The listing builds one solid part. Answer for the finished solid, in the listing's coordinates (mm). Face numbers are marked on the shaded views. A direction names the side the tool comes from. Give positions to 0.01 mm unless a question says otherwise; leave off trailing zeros. Write each loop counter-clockwise with the first axis right and the second up, starting at its lowest first coordinate (ties: lowest second). Pieces come first, ordered by that corner, then holes. Notation, with made-up numbers: (-13, 52.5) - (20, 52.5) arc R23 cw to (20, 86.5) - close; hole circle Ø1 at (-4, 86.25). An arc over 180 degrees is marked (long way). Answer as CSV lines item,"result". Start each with the question number.
(1) For the marked faces 1, 2 and 3, determine the directions among +Z, -Z, +X, -X, +Y, -Y from which every point of the face is accessible in a straight line to the end or side of a thin tool.
(2) Each of these flat-tipped pins is pushed along its axis until it touches: pin 1 Ø5 at (y, z) = (30.5, 10.5) entering from +X; pin 2 Ø1.3 at (x, y) = (-1, 28) entering from +Z; pin 3 Ø5 at (y, z) = (13.5, 3) entering from -X. Where does it stop, or does it pass through?
(3) Find section D-D (y = 7). Write down the section's boundary in (x, z), then the cut area to 3 significant figures.
(4) Find section B-B (x = 25). Write down the section's boundary in (y, z).
(5) Straight lines are drawn through the part: probe 1 along Y at (x, z) = (-25, 6.25); probe 2 along Y at (x, z) = (0, 7.5); probe 3 along Y at (x, z) = (-30, 6). For each, find the intervals that lie inside material, in ascending order.
(6) Find section C-C (z = 5.5). Write down the section's boundary in (x, y).
(7) Find section A-A (y = 0). Write down the section's boundary in (x, z).
from build123d import *

# Parameters (mm, degrees)
SKETCH1_W           = 71
SKETCH1_H           = 25.6
BOSS_EXTRUDE1_DEPTH = 10
BOSS_EXTRUDE2_DEPTH = 14
FILLET1_R           = 4
CHAMFER1_START      = -22.201998907
CHAMFER1_OUTLINE_W  = 14.611297
CHAMFER1_OUTLINE_H  = 10
CHAMFER1_DEPTH      = 3.757366646
CHAMFER2_START      = 18.444632261
CHAMFER2_OUTLINE_W  = 14.611297
CHAMFER2_OUTLINE_H  = 10
CHAMFER2_DEPTH      = 3.757366646
FILLET3_R           = 2
SKETCH5_R           = 2.35
CUT_EXTRUDE1_DEPTH  = 14
FILLET4_R           = 2
SKETCH6_R           = 2.15
CUT_EXTRUDE2_DEPTH  = 13


with BuildPart() as part:
    # Sketch1 → Boss-Extrude1 (new body)
    with BuildSketch(Plane.XY):
        Rectangle(SKETCH1_W, SKETCH1_H)
    extrude(amount=BOSS_EXTRUDE1_DEPTH)

    # Sketch3 → Boss-Extrude2 (add)
    with BuildSketch(Plane.XY):
        with BuildLine():
            Line((-17, 12.8), (17, 12.8))
            Line((17, 12.8), (17, 27.1))
            ThreePointArc((17, 27.1), (0, 44.1), (-17, 27.1))
            Line((-17, 27.1), (-17, 12.8))
        make_face()
    extrude(amount=BOSS_EXTRUDE2_DEPTH)

    # Fillet1
    fillet1_edges = [part.edges().sort_by_distance(p)[0] for p in [
        (0, 12.8, 10),
    ]]
    fillet(fillet1_edges, radius=FILLET1_R - 0.0001)  # a hair under: the kernel refuses the full size

    # Chamfer1: read off the stored shape, not the designer's step
    # Chamfer1 outline → Chamfer1 (add)
    with BuildSketch(Plane(origin=(0, 0, 0), x_dir=(0.2053205817495901, 0.9786947730063801, 0), z_dir=(0.9786947730063802, -0.20532058174959006, 0)).offset(CHAMFER1_START)):
        with Locations((15.726529959, 5)):
            Rectangle(CHAMFER1_OUTLINE_W, CHAMFER1_OUTLINE_H)
    extrude(amount=CHAMFER1_DEPTH)

    # Chamfer2: read off the stored shape, not the designer's step
    # Chamfer2 outline → Chamfer2 (add)
    with BuildSketch(Plane(origin=(0, 0, 0), x_dir=(-0.2053205817495901, 0.9786947730063801, 0), z_dir=(0.9786947730063802, 0.20532058174959006, 0)).offset(CHAMFER2_START)):
        with Locations((15.726529959, 5)):
            Rectangle(CHAMFER2_OUTLINE_W, CHAMFER2_OUTLINE_H)
    extrude(amount=CHAMFER2_DEPTH)

    # Fillet3
    fillet3_edges = [part.edges().sort_by_distance(p)[0] for p in [
        (-20.000000001, 12.8, 5),
        (20.000000001, 12.8, 5),
        (35.5, -12.8, 5),
        (-35.5, -12.8, 5),
        (-35.5, 12.8, 5),
        (35.5, 12.8, 5),
    ]]
    fillet(fillet3_edges, radius=FILLET3_R)

    # Sketch5 → Cut-Extrude1 (cut)
    with BuildSketch(Plane.XY.offset(10)):
        with Locations((-25, 0)):
            Circle(SKETCH5_R)
        with Locations(Location((25, 0, 0), (0, 0, 180))):
            Circle(SKETCH5_R)
    extrude(amount=-CUT_EXTRUDE1_DEPTH, mode=Mode.SUBTRACT)

    # Fillet4
    fillet4_edges = [part.edges().sort_by_distance(p)[0] for p in [
        (-27.35, 0, 0),
        (27.35, 0, 0),
        (0, 44.1, 0),
        (-18.333284039, 20.744679418, 0),
        (27.561978811, 12.8, 0),
        (35.5, 0, 0),
        (0, -12.8, 0),
        (-35.5, 0, 0),
        (-27.561978811, 12.8, 0),
        (18.333284039, 20.744679418, 0),
        (-34.914213562, 12.214213562, 0),
        (-34.914213562, -12.214213562, 0),
        (34.914213562, -12.214213562, 0),
        (34.914213562, 12.214213562, 0),
        (-20.363259865, 13.247376039, 0),
        (20.363259865, 13.247376039, 0),
    ]]
    fillet(fillet4_edges, radius=FILLET4_R)

    # Sketch6 → Cut-Extrude2 (cut)
    with BuildSketch(Plane.XY.offset(14)):
        with Locations((0, 27.1)):
            Circle(SKETCH6_R)
    extrude(amount=-CUT_EXTRUDE2_DEPTH, mode=Mode.SUBTRACT)


solid = part.part
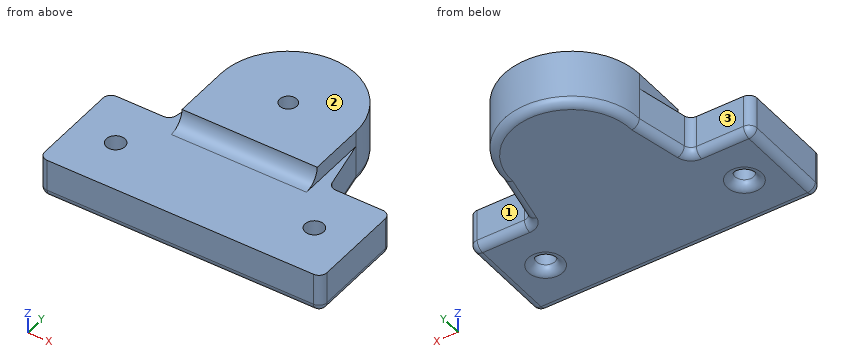
Result set:
1,face 1,"+Z, -Z, +X, +Y"
1,face 2,"+Z, +X, -X, +Y, -Y"
1,face 3,"+Z, -Z, -X, +Y"
2,pin 1,"x = 16.98"
2,pin 2,"z = 1"
2,pin 3,"x = -35.49"
3,outline,"(-35.5, 2) arc R2 ccw to (-33.5, 0) - (33.5, 0) arc R2 ccw to (35.5, 2) - (35.5, 10) - (-35.5, 10) - close"
3,area,"708 mm^2"
4,outline,"(-12.8, 2) arc R2 ccw to (-10.8, 0) - (-4.35, 0) arc R2 ccw to (-2.35, 2) - (-2.35, 10) - (-12.8, 10) - close; (2.35, 2) arc R2 ccw to (4.35, 0) - (10.8, 0) arc R2 ccw to (12.8, 2) - (12.8, 10) - (2.35, 10) - close"
5,probe 1,"-12.8 to -2.35, 2.35 to 12.8"
5,probe 2,"-12.8 to 24.95, 29.25 to 44.1"
5,probe 3,"-12.8 to 12.8"
6,outline,"(-35.5, -10.8) arc R2 ccw to (-33.5, -12.8) - (33.5, -12.8) arc R2 ccw to (35.5, -10.8) - (35.5, 10.8) arc R2 ccw to (33.5, 12.8) - (21.62, 12.8) arc R2 cw to (19.67, 14.39) - (17, 27.1) arc R17 ccw to (-17, 27.1) - (-19.67, 14.39) arc R2 cw to (-21.62, 12.8) - (-33.5, 12.8) arc R2 ccw to (-35.5, 10.8) - close; hole circle Ø4.7 at (-25, 0); hole circle Ø4.3 at (0, 27.1); hole circle Ø4.7 at (25, 0)"
7,outline,"(-35.5, 2) arc R2 ccw to (-33.5, 0) - (-29.35, 0) arc R2 ccw to (-27.35, 2) - (-27.35, 10) - (-35.5, 10) - close; (-22.65, 2) arc R2 ccw to (-20.65, 0) - (20.65, 0) arc R2 ccw to (22.65, 2) - (22.65, 10) - (-22.65, 10) - close; (27.35, 2) arc R2 ccw to (29.35, 0) - (33.5, 0) arc R2 ccw to (35.5, 2) - (35.5, 10) - (27.35, 10) - close"
